Here's how the part is built. I have some questions about the finished solid (model axes, mm). A direction names the side the tool comes from. Give positions to 0.01 mm unless a question says otherwise; leave off trailing zeros. Order: outer loops, then holes, each group sorted by start corner. A loop starts at its lowest first (then second) coordinate and runs counter-clockwise, first axis right, second up. Notation, with made-up numbers: (-12, -15) - (-5, -15) arc R36 ccw to (-5, 20) - close; hole circle Ø3 at (45, -12.5). An arc over 180 degrees is marked (long way). One line per question, with ' | ' between items.
from build123d import *

# Parameters (mm, degrees)
F1_DEPTH     = 16
F2_R         = 3
F3_R         = 1.5
F4_DEPTH     = 2
F5_T         = 1.5
F5_T3_DEPTH  = 5
F5_T5_DEPTH  = 6.5
F5_T7_DEPTH  = 32
F5_T9_DEPTH  = 29
F5_T12_ANGLE = 90.000000001
F5_T14_ANGLE = 90.000000001
F7_DEPTH     = 13.001
F6_R         = 2.5
F6_R_2       = 1.75
F8_DEPTH     = 1.5
F9_R         = 1


# Not quite as in the source:
# - a shell that OpenCascade refuses in one call is made with other operations: the cavity is built on its own and cut out


with BuildPart() as f1:
    # F0 (on Right) → F1 (new body, symmetric)
    with BuildSketch(Plane.YZ):
        Polygon((12, -4.5), (-4, 6.5), (-12, 6.5), (-12, -6.5), (12, -6.5), align=None)
    extrude(amount=F1_DEPTH, both=True)

    # F2
    f2_edges = [f1.edges().sort_by_distance(p)[0] for p in [
        (16, 12, -5.5),
        (-16, 12, -5.5),
        (16, 4, 1),
        (-16, 4, 1),
    ]]
    fillet(f2_edges, radius=F2_R)

    # F3 (on face) → F4 (cut)
    with BuildSketch(Plane(origin=(0, 0, -6.5), x_dir=(1, 0, 0), z_dir=(0, 0, -1))):
        with BuildLine():
            ThreePointArc((13, -10.5), (14.0606601718, -10.0606601718), (14.5, -9))
            Line((14.5, -9), (14.5, -5.5))
            Line((14.5, -5.5), (-14.5, -5.5))
            Line((-14.5, -5.5), (-14.5, -9))
            ThreePointArc((-14.5, -9), (-14.0606601718, -10.0606601718), (-13, -10.5))
            Line((-13, -10.5), (13, -10.5))
        make_face()
        with Locations((-8, -8)):
            Circle(F3_R, mode=Mode.SUBTRACT)
        with Locations((0, -8)):
            Circle(F3_R, mode=Mode.SUBTRACT)
        with Locations((8, -8)):
            Circle(F3_R, mode=Mode.SUBTRACT)
    extrude(amount=-F4_DEPTH, mode=Mode.SUBTRACT)

    # F5: shell of thickness 1.5, made by hand


with BuildPart() as f5_core1:
    # F5_t2: copy of F1
    add(f1.part)

    # the walls: a layer under each face that stays
    f5_faces = [f5_core1.faces().sort_by_distance(p)[0] for p in [
        (0, 4, 1),
        (0, -8, 6.5),
        (-15.1213203436, 1.7042929957, 1.5119940115),
        (15.1213203436, 1.7042929957, 1.5119940115),
        (0, 12, -5.5),
        (-16, -1.5, 0),
        (16, -1.5, 0),
        (-15.1213203436, 11.1213203436, -5.5),
        (15.1213203436, 11.1213203436, -5.5),
        (14.0606601718, 10.0606601718, -5.5),
        (14.5, 7.25, -5.5),
        (0, 5.5, -5.5),
        (-14.5, 7.25, -5.5),
        (-14.0606601718, 10.0606601718, -5.5),
        (0, 10.5, -5.5),
        (-9.6666666667, 9.6666666667, -4.5),
        (-8, 8, -6.5),
        (0, 8, -6.5),
        (8, 8, -6.5),
    ]]
    thicken(f5_faces, amount=-F5_T, mode=Mode.SUBTRACT)

    # F5_s4 → F5_t3 (cut)
    with BuildSketch(Plane.XY.offset(-8)):
        Polygon((14.485, 5.515), (16, 5.5), (16, 4), (14.5, 4), align=None)
        Polygon((-14.485, 5.515), (-14.5, 4), (-16, 4), (-16, 5.5), align=None)
    extrude(amount=F5_T3_DEPTH, mode=Mode.SUBTRACT)

    # F5_s6 → F5_t5 (cut)
    with BuildSketch(Plane.XZ.offset(-10.5)):
        Polygon((14.485, -4.515), (16, -4.5), (16, -3), (14.5, -3), align=None)
        Polygon((-14.485, -4.515), (-16, -4.5), (-16, -3), (-14.5, -3), align=None)
    extrude(amount=F5_T5_DEPTH, mode=Mode.SUBTRACT)

    # F5_s8 → F5_t7 (cut)
    with BuildSketch(Plane.YZ.offset(-16)):
        Polygon((5.515, -4.515), (4, -4.5), (4, -3), (5.5, -3), align=None)
    extrude(amount=F5_T7_DEPTH, mode=Mode.SUBTRACT)

    # F5_s10 → F5_t9 (cut)
    with BuildSketch(Plane.YZ.offset(-14.5)):
        Polygon((10.485, -4.515), (12, -4.5), (12, -3), (10.5, -3), align=None)
    extrude(amount=F5_T9_DEPTH, mode=Mode.SUBTRACT)

    # F5_s11 → F5_t12 (revolve, cut)
    with BuildSketch(Plane.YZ.offset(13)):
        Polygon((10.485, -4.515), (12, -4.5), (12, -3), (10.5, -3), align=None)
    revolve(axis=Axis((13, 9, -4.5), (0, 0, -1)), revolution_arc=F5_T12_ANGLE, mode=Mode.SUBTRACT)

    # F5_s13 → F5_t14 (revolve, cut)
    with BuildSketch(Plane.XZ.offset(-9)):
        Polygon((-14.485, -4.515), (-16, -4.5), (-16, -3), (-14.5, -3), align=None)
    revolve(axis=Axis((-13, 9, -4.5), (0, 0, -1)), revolution_arc=F5_T14_ANGLE, mode=Mode.SUBTRACT)

    # F5_s15 → F5_t16 (revolve, cut)
    with BuildSketch(Plane.XZ.offset(-8)):
        Polygon((-6.485, -4.515), (-6.5, -3), (-8, -3), (-8, -4.5), align=None)
    revolve(axis=Axis((-8, 8, -4.5), (0, 0, -1)), mode=Mode.SUBTRACT)

    # F5_s17 → F5_t18 (revolve, cut)
    with BuildSketch(Plane.XZ.offset(-8)):
        Polygon((1.515, -4.515), (1.5, -3), (0, -3), (0, -4.5), align=None)
    revolve(axis=Axis((0, 8, -4.5), (0, 0, -1)), mode=Mode.SUBTRACT)

    # F5_s19 → F5_t20 (revolve, cut)
    with BuildSketch(Plane.XZ.offset(-8)):
        Polygon((9.515, -4.515), (9.5, -3), (8, -3), (8, -4.5), align=None)
    revolve(axis=Axis((8, 8, -4.5), (0, 0, -1)), mode=Mode.SUBTRACT)


with BuildPart() as f1_1:
    add(f1.part)

    # what is left inside the walls is the cavity
    f5_cavity = [f5_core1.part.solids().sort_by_distance(p)[0] for p in [
        (-4.833333, -4, -6.485),
    ]]
    add(f5_cavity, mode=Mode.SUBTRACT)

    # F6 (on face) → F7 (cut, through all)
    with BuildSketch(Plane.XY.offset(6.5)):
        with BuildLine():
            Line((9.5, -5), (-9.5, -5))
            Line((-9.5, -5), (-9.5, -8))
            ThreePointArc((-9.5, -8), (-10.6715728753, -10.8284271247), (-13.5, -12))
            Line((-13.5, -12), (13.5, -12))
            ThreePointArc((13.5, -12), (10.6715728753, -10.8284271247), (9.5, -8))
            Line((9.5, -8), (9.5, -5))
        make_face()
    extrude(amount=-F7_DEPTH, mode=Mode.SUBTRACT)

    # F6 (on face) → F8 (join)
    with BuildSketch(Plane.XY.offset(6.5)):
        with Locations((-12, -8)):
            Circle(F6_R)
        with Locations((-12, -8)):
            Circle(F6_R_2, mode=Mode.SUBTRACT)
        with BuildLine():
            ThreePointArc((14.5, -8), (12, -5.5), (9.5, -8))
            ThreePointArc((9.5, -8), (12, -10.5), (14.5, -8))
        make_face()
        with Locations((12, -8)):
            Circle(F6_R_2, mode=Mode.SUBTRACT)
    extrude(amount=F8_DEPTH)

    # F9
    f9_edges = [f1_1.edges().sort_by_distance(p)[0] for p in [
        (15.25, -12, -6.5),
        (-15.25, -12, -6.5),
    ]]
    fillet(f9_edges, radius=F9_R)


solid = f1_1.part
1) On a 3-axis mill with a long thin cutter (end or side, diameter ignored), from which of +Z, -Z, +X, -X, +Y, -Y can I reach the whole of each face in a straight line? I mean faces 1 (the face through (0, 8, -6.5)), 2 (the face through (-8.325, 9.464, -5.514)), 3 (the face through (0, 12, -6)), 4 (the face through (3.4, -4.8, 5)), 5 (the face through (13.617, -8.67, 7.24)). Say none if no direction works.
Model answer:
face 1: -Z, +X, -X, +Y, -Y | face 2: -Z | face 3: +Z, -Z, +X, -X, +Y | face 4: -Z, -Y | face 5: +Z
2) I want a section at A-A (x = 0). List the corners of the cut face in (y, z) for me.
Model answer:
outline: (-5, 5) - (-4.47, 5) - (7.17, -3) - (4, -3) - (4, -6.5) - (5.5, -6.5) - (5.5, -4.5) - (6.5, -4.5) - (6.5, -6.5) - (9.5, -6.5) - (9.5, -4.5) - (10.5, -4.5) - (10.5, -6.5) - (12, -6.5) - (12, -4.5) - (-4, 6.5) - (-5, 6.5) - close
3) I want a section at B-B (z = 7.25). List the corners of the cut face in (x, y) for me.
Model answer:
outline: circle Ø5 at (-12, -8); circle Ø5 at (12, -8); hole circle Ø3.5 at (-12, -8); hole circle Ø3.5 at (12, -8)
4) I'm going to push flat-ended pins straight in: P1, Ø3, axis at x = -3.5, y = 8.5, coming from the -Z side; P2, Ø1.8, axis at x = -1.5, z = -4, coming from the -Y side; P3, Ø1.2, axis at y = -6, z = 5.5, coming from the -X side. Where does each tip first touch, or does it pass through?
Model answer:
P1: stops at z = -4.5 | P2: stops at y = 4 | P3: stops at x = -15.97
5) Thinking about a two-plate mould opening in X: for faces 6 (the face through (-15.26, -11.715, -6.199)), 7 (the face through (16, -4, -1)), 8 (the face through (10.703, -10.859, 5.76)), 9 (the face through (0, 10, -4.5)), which applies, +X half, -X half, draft (parallel to the pull), parting line (faces both ways), or undercut?
Model answer:
face 6: draft | face 7: +X half | face 8: undercut | face 9: undercut
6) I want a section at C-C (x = 12). List the corners of the cut face in (y, z) for me, plus the area to 3 significant figures.
Model answer:
outline: (-11.71, 5) - (-4.47, 5) - (7.17, -3) - (4, -3) - (4, -6.5) - (5.5, -6.5) - (5.5, -4.5) - (10.5, -4.5) - (10.5, -6.5) - (12, -6.5) - (12, -4.5) - (-4, 6.5) - (-5.5, 6.5) - (-5.5, 8) - (-6.25, 8) - (-6.25, 6.5) - (-9.75, 6.5) - (-9.75, 8) - (-10.5, 8) - (-10.5, 6.5) - (-11.71, 6.5) - close | area: 53.0 mm2
7) Please list where these lines run through material, in increasing order: L1, parallel to Y at x = -10, z = -4.75; L2, parallel to X at y = -8.25, z = -2; L3, parallel to X at y = 7, z = -5.5.
Model answer:
L1: y = 4 to 5.5, 10.5 to 12 | L2: x = -16 to -14.5, 14.5 to 16 | L3: x = -16 to -14.5, -9.12 to -6.88, -1.12 to 1.12, 6.88 to 9.12, 14.5 to 16
